Input: part model. Units: mm. Frame: model coordinates. Face numbers are marked on the shaded views. Round coordinates to 2 decimals unless told otherwise and drop trailing zeros. Loops run counter-clockwise (first coordinate to the right, second up) from the corner with the lowest first, then second, coordinate; pieces in that order, holes last. Notation, with made-up numbers: M 30,68.25 L 47,68.25 A26 cw 47,85.25 Z; hole C 25,23.5 d7. An arc over 180 degrees is marked long. Put each result on its own line as item: value. Start each with the question number.
1) Draft query along X for the marked faces 1, 2, 3 and 4. Return one class per face: +X half, -X half, draft (parallel to the pull), parting line (faces both ways), or undercut.
2) Pin query (flat end, axial travel): pin 1 (1.5 mm diameter, centred on x = -12.5, z = 1.5, fed in from +Y); pin 2 (0.9 mm diameter, centred on x = -13.5, z = 1, fed in from -Y). Return the tip coordinate at first contact, or that it passes through.
3) Section B-B on y = -2.6. Output: boundary loops of the cut face in (x, z), plus the area to 3 significant figures.
4) Section C-C on x = -4.25. Output: boundary loops of the cut face in (y, z).
5) Section A-A on z = 1.6. Output: boundary loops of the cut face in (x, y), plus the area to 3 significant figures.
6) Section D-D on y = -0.3. Output: boundary loops of the cut face in (x, z).
7) Line query: probe 1 along Y at (x, z) = (-23, 1); probe 2 along X at (y, z) = (-3.3, 1); probe 3 along X at (y, z) = (-3.05, 0.25). Output: solid intervals per line, ascending.
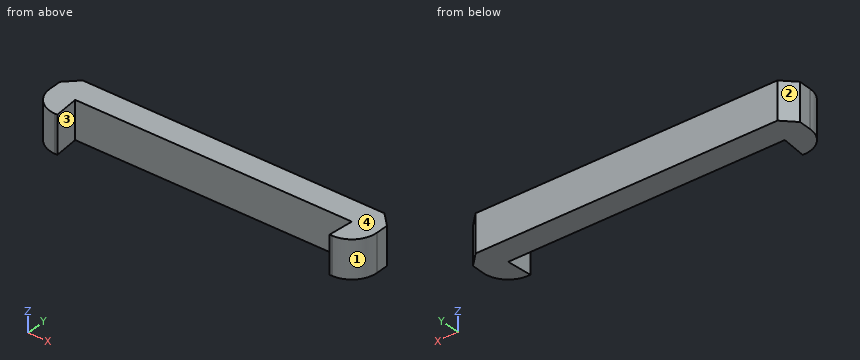
Autodesk Inventor part; units mm, degrees
ref_plane "YZ Plane" through (0, 0, 0) normal (1, 0, 0) x (0, 1, 0)
ref_plane "XZ Plane" through (0, 0, 0) normal (0, 1, 0) x (-1, 0, 0)
ref_plane "XY Plane" through (0, 0, 0) normal (0, 0, 1) x (1, 0, 0)
sketch "Sketch2" plane through (0, 0, 0) normal (0, 0, 1) x (1, 0, 0)
  line L0 (0, 0) -> (-25, 0)
  line L1 (-25, 0) -> (-25, -2)
  line L2 (-25, -2) -> (0, -2)
  line L3 (0, -2) -> (0, 0)
  line L4 (-25.5, 0) -> (-23.5, 0)
  line L5 (-23.5, 0) -> (-23.5, -4)
  line L6 (-23.5, -4) -> (-25.5, -4)
  line L7 (-25.5, -4) -> (-25.5, 0)
  line L8 (0.5, 0) -> (-1.5, 0)
  line L9 (-1.5, 0) -> (-1.5, -4)
  line L10 (-1.5, -4) -> (0.5, -4)
  line L11 (0.5, -4) -> (0.5, 0)
  point P0 (-23.5, -2)
  point P1 (-1.5, -2)
  dimension "d0" = 25
  dimension "d1" = 2
  dimension "d2" = 2
  dimension "d3" = 4
  dimension "d4" = 2
  dimension "d5" = 4
extrude "Extrusion1" add sketch "Sketch2" along normal blind 3
chamfer "Chamfer1" distance 1 angle 45 2 edges at (-25.5, 0, 1.5) (0.5, 0, 1.5)
draft "FaceDraft1" angle -5 pull direction (0, -1, 0) faces at (-23.5, -3.3333, 1) fixed edges at (-23.5, -2, 1.5)
draft "FaceDraft2" angle -5 pull direction (0, -1, 0) faces at (-1.5, -2.6667, 1) fixed edges at (-1.5, -2, 1.5)
fillet "Fillet1" radius 2 2 edges at (-25.5, -4, 1.5) (0.5, -4, 1.5)
properties part number "Clip"
Geometry results:
1. face 1: +X half
1. face 2: -X half
1. face 3: undercut
1. face 4: draft
2. pin 1: stops at y = 0
2. pin 2: stops at y = -2
3. outline: M -25.41,0 L -23.45,0 L -23.45,3 L -25.41,3 Z; M -1.55,0 L 0.41,0 L 0.41,3 L -1.55,3 Z
3. area: 11.8 mm²
4. outline: M -2,0 L 0,0 L 0,3 L -2,3 Z
5. outline: M -25.5,-2 A2 ccw -23.5,-4 L -23.33,-4 L -23.5,-2 L -1.5,-2 L -1.67,-4 L -1.5,-4 A2 ccw 0.5,-2 L 0.5,-1 L -0.5,0 L -24.5,0 L -25.5,-1 Z
5. area: 57.6 mm²
6. outline: M -24.8,0 L -0.2,0 L -0.2,3 L -24.8,3 Z
7. probe 1: y = -2 to 0
7. probe 2: x = -25.02 to -23.39, -1.61 to 0.02
7. probe 3: x = -25.2 to -23.41, -1.59 to 0.2
